```python
from build123d import *

# Parameters (mm, degrees)
SKETCH1_W           = 50
SKETCH1_H           = 40
BOSS_EXTRUDE1_DEPTH = 10
SKETCH5_W           = 6
SKETCH5_H           = 5
BOSS_EXTRUDE3_DEPTH = 10
SKETCH6_R           = 1.25
CUT_EXTRUDE1_DEPTH  = 20
SKETCH8_W           = 10
SKETCH8_H           = 40
CUT_EXTRUDE2_DEPTH  = 25
SKETCH12_W          = 5
SKETCH12_H          = 5
BOSS_EXTRUDE5_DEPTH = 10
SKETCH13_R          = 1.25
CUT_EXTRUDE4_DEPTH  = 10
SKETCH14_R          = 2.5
CUT_EXTRUDE5_DEPTH  = 10
CUT_EXTRUDE6_DEPTH  = 22
CUT_EXTRUDE7_DEPTH  = 30
CUT_EXTRUDE8_DEPTH  = 30
SCALE1_SCALE        = 2
SKETCH19_W          = 172.616714004
SKETCH19_H          = 129.336721571
SKETCH19_W_2        = 100
SKETCH19_H_2        = 80
CUT_EXTRUDE9_DEPTH  = 20
SKETCH20_W          = 100
SKETCH20_H          = 80
CUT_EXTRUDE10_DEPTH = 10
BOSS_EXTRUDE6_DEPTH = 20
SKETCH22_W          = 5
SKETCH22_H          = 10
CUT_EXTRUDE11_DEPTH = 50


with BuildPart() as part:
    # Sketch1 → Boss-Extrude1 (new body)
    with BuildSketch(Plane(origin=(669.84184187, 0, 0), x_dir=(1, 0, 0), z_dir=(0, 0, 1))):
        with Locations((-671.310344828, 437.637931034)):
            Rectangle(SKETCH1_W, SKETCH1_H)
    boss_extrude1 = extrude(amount=BOSS_EXTRUDE1_DEPTH)

    # Sketch5 → Boss-Extrude3 (add)
    with BuildSketch(Plane(origin=(23.531497042, 0, 0), x_dir=(0, 0, -1), z_dir=(1, 0, 0))):
        with Locations((-5, 442.637931034)):
            Rectangle(SKETCH5_W, SKETCH5_H)
        with Locations((-5, 432.637931034)):
            Rectangle(SKETCH5_W, SKETCH5_H)
    boss_extrude3 = extrude(amount=BOSS_EXTRUDE3_DEPTH)

    # Sketch6 → Cut-Extrude1 (cut)
    with BuildSketch(Plane(origin=(669.84184187, 445.137931034, 0), x_dir=(1, 0, 0), z_dir=(0, 1, 0))):
        with Locations(Location((-641.310344828, -5, 0), (0, 0, 180))):
            Circle(SKETCH6_R)
    cut_extrude1 = extrude(amount=-CUT_EXTRUDE1_DEPTH, mode=Mode.SUBTRACT)

    # Sketch8 → Cut-Extrude2 (cut)
    with BuildSketch(Plane.ZY.offset(26.468502958)):
        with Locations((5, 437.637931034)):
            Rectangle(SKETCH8_W, SKETCH8_H)
    extrude(amount=-CUT_EXTRUDE2_DEPTH, mode=Mode.SUBTRACT)

    # Mirror1: Boss-Extrude1, Boss-Extrude3, Cut-Extrude1 across plane
    add(boss_extrude1.mirror(Plane(origin=(-1.468502958, 0, 0), x_dir=(0, 0, 1), z_dir=(1, 0, 0))))
    add(boss_extrude3.mirror(Plane(origin=(-1.468502958, 0, 0), x_dir=(0, 0, 1), z_dir=(1, 0, 0))))
    add(cut_extrude1.mirror(Plane(origin=(-1.468502958, 0, 0), x_dir=(0, 0, 1), z_dir=(1, 0, 0))), mode=Mode.SUBTRACT)

    # Sketch12 → Boss-Extrude5 (add)
    with BuildSketch(Plane(origin=(0, 457.637931034, 0), x_dir=(1, 0, 0), z_dir=(0, 1, 0))):
        with Locations((-1.468502958, -5)):
            Rectangle(SKETCH12_W, SKETCH12_H)
    extrude(amount=BOSS_EXTRUDE5_DEPTH)

    # Sketch13 → Cut-Extrude4 (cut)
    with BuildSketch(Plane(origin=(1.031497042, 0, 0), x_dir=(0, 0, -1), z_dir=(1, 0, 0))):
        with Locations((-5, 462.637931034)):
            Circle(SKETCH13_R)
    extrude(amount=-CUT_EXTRUDE4_DEPTH, mode=Mode.SUBTRACT)

    # Sketch14 → Cut-Extrude5 (cut)
    with BuildSketch(Plane.XY.offset(10)):
        with Locations((-16.468502958, 447.637931034)):
            Circle(SKETCH14_R)
        with Locations((-16.468502958, 427.637931034)):
            Circle(SKETCH14_R)
        with Locations((13.531497042, 447.637931034)):
            Circle(SKETCH14_R)
        with Locations((13.531497042, 427.637931034)):
            Circle(SKETCH14_R)
    extrude(amount=-CUT_EXTRUDE5_DEPTH, mode=Mode.SUBTRACT)

    # Sketch15 → Cut-Extrude6 (cut)
    with BuildSketch(Plane(origin=(0, 445.137931034, 0), x_dir=(1, 0, 0), z_dir=(0, 1, 0))):
        with BuildLine():
            Line((33.531497042, -2), (28.531497042, -2))
            ThreePointArc((28.531497042, -2), (30.652817386, -2.878679656), (31.531497042, -5))
            ThreePointArc((31.531497042, -5), (30.652817386, -7.121320344), (28.531497042, -8))
            Line((28.531497042, -8), (33.531497042, -8))
            Line((33.531497042, -8), (33.531497042, -2))
        make_face()
    extrude(amount=-CUT_EXTRUDE6_DEPTH, mode=Mode.SUBTRACT)

    # Sketch17 → Cut-Extrude7 (cut)
    with BuildSketch(Plane(origin=(0, 445.137931034, 0), x_dir=(1, 0, 0), z_dir=(0, 1, 0))):
        with BuildLine():
            Line((-36.468502958, -8), (-31.468502958, -8))
            ThreePointArc((-31.468502958, -8), (-34.468502958, -5), (-31.468502958, -2))
            Line((-31.468502958, -2), (-36.468502958, -2))
            Line((-36.468502958, -2), (-36.468502958, -8))
        make_face()
    extrude(amount=-CUT_EXTRUDE7_DEPTH, mode=Mode.SUBTRACT)

    # Sketch18 → Cut-Extrude8 (cut)
    with BuildSketch(Plane(origin=(1.031497042, 0, 0), x_dir=(0, 0, -1), z_dir=(1, 0, 0))):
        with BuildLine():
            Line((-7.5, 467.637931034), (-7.5, 462.637931034))
            ThreePointArc((-7.5, 462.637931034), (-5, 465.137931034), (-2.5, 462.637931034))
            Line((-2.5, 462.637931034), (-2.5, 467.637931034))
            Line((-2.5, 467.637931034), (-7.5, 467.637931034))
        make_face()
    extrude(amount=-CUT_EXTRUDE8_DEPTH, mode=Mode.SUBTRACT)


with BuildPart() as part_1:
    # Scale1: scaled about (-1.468502958, 437.810556227, 5)
    add(part.part.scale(SCALE1_SCALE).moved(Location((1.468502958, -437.810556227, -5))))

    # Sketch19 → Cut-Extrude9 (cut)
    with BuildSketch(Plane.XY.offset(15)):
        with Locations((2.170441993, 437.623617036)):
            Rectangle(SKETCH19_W, SKETCH19_H)
        with Locations((-1.468502958, 437.465305842)):
            Rectangle(SKETCH19_W_2, SKETCH19_H_2, mode=Mode.SUBTRACT)
    extrude(amount=-CUT_EXTRUDE9_DEPTH, mode=Mode.SUBTRACT)

    # Sketch20 → Cut-Extrude10 (cut)
    with BuildSketch(Plane.XY.offset(15)):
        with Locations((-1.468502958, 437.465305842)):
            Rectangle(SKETCH20_W, SKETCH20_H)
    extrude(amount=-CUT_EXTRUDE10_DEPTH, mode=Mode.SUBTRACT)

    # Sketch21 → Boss-Extrude6 (add)
    with BuildSketch(Plane.XY.offset(5)):
        Polygon((-11.468502958, 477.465305842), (-21.468502958, 477.465305842), (-21.468502958, 397.465305842), (-11.468502958, 397.465305842), (-11.468502958, 464.619479755), align=None)
        Polygon((18.531497042, 477.465305842), (8.531497042, 477.465305842), (8.531497042, 471.588870089), (8.531497042, 397.465305842), (18.531497042, 397.465305842), align=None)
    extrude(amount=BOSS_EXTRUDE6_DEPTH)

    # Sketch22 → Cut-Extrude11 (cut)
    with BuildSketch(Plane.ZY.offset(21.468502958)):
        with Locations((17.5, 462.465305842)):
            Rectangle(SKETCH22_W, SKETCH22_H)
        with Locations((17.5, 412.465305842)):
            Rectangle(SKETCH22_W, SKETCH22_H)
    extrude(amount=-CUT_EXTRUDE11_DEPTH, mode=Mode.SUBTRACT)


solid = part_1.part
```
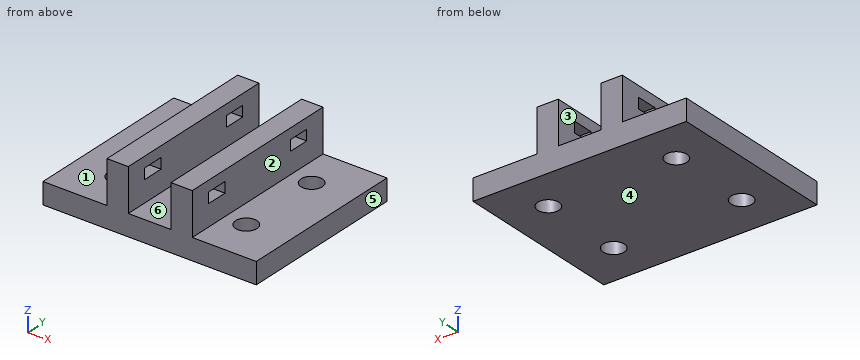
The listing builds one solid part. Answer for the finished solid, in the listing's coordinates (mm). Face numbers are marked on the shaded views. A direction names the side the tool comes from. Coordinates: 2 decimals unless noted, no trailing zeros. Order: outer loops, then holes, each group sorted by start corner. A loop starts at its lowest first (then second) coordinate and runs counter-clockwise, first axis right, second up. Notation, with made-up numbers: M 44.25,77.25 L 54.25,77.25 A24 cw 54.25,93.25 Z; hole C -14,59 d11. An arc over 180 degrees is marked long. Answer as a JSON object with one key per item and string values. Group by question number.
1. Section D-D on y = 446.5 is taken. Write down the section's boundary in (x, z).
2. Straight lines are drawn through the part: line 1 (X direction, y = 428, z = 23.5); line 2 (Z direction, x = -38.5, y = 418). For each, find the intervals that lie inside material, in ascending order.
3. Section C-C on y = 456 is taken. Write down the section's boundary in (x, z).
4. Section A-A on x = 10.5 is taken. Write down the section's boundary in (y, z), then the cut area to 3 significant figures.
5. Flat-ended cylindrical pins translate along their axes: P1, Ø16, axis at x = -5.5, y = 421, coming from the +Z side; P2, Ø1, axis at x = 7.5, y = 462.5, coming from the +Z side; P3, Ø4, axis at y = 434.5, z = 7.5, coming from the -X side; P4, Ø16, axis at y = 421, z = 15, coming from the +X side. Find the tip coordinate at first contact, or state that the pin passes through.
6. Determine the mould class of the marked faces 4, 5 and 6 for opening direction X: released by +X, released by -X, zero draft, split by the parting line, or undercut.
7. Section B-B on z = 11 is taken. Write down the section's boundary in (x, y).
8. A tool of negligible diameter and unlimited length cuts with its end or side. For the marked faces 1, 2 and 3, from which of +Z, -Z, +X, -X, +Y, -Y can it reach the whole face along a straight path? Write none if from no direction.
Values follow:
{
 "1": {"outline": "M -51.47,-5 L 48.53,-5 L 48.53,5 L 18.53,5 L 18.53,25 L 8.53,25 L 8.53,5 L -11.47,5 L -11.47,25 L -21.47,25 L -21.47,5 L -51.47,5 Z"},
 "2": {"line 1": "-21.47 to -11.47, 8.53 to 18.53", "line 2": "-5 to 5"},
 "3": {"outline": "M -51.47,-5 L -36.25,-5 L -36.25,5 L -51.47,5 Z; M -26.69,-5 L 23.75,-5 L 23.75,5 L 18.53,5 L 18.53,25 L 8.53,25 L 8.53,5 L -11.47,5 L -11.47,25 L -21.47,25 L -21.47,5 L -26.69,5 Z; M 33.31,-5 L 48.53,-5 L 48.53,5 L 33.31,5 Z"},
 "4": {"outline": "M 397.47,-5 L 477.47,-5 L 477.47,25 L 397.47,25 Z; hole M 407.47,15 L 417.47,15 L 417.47,20 L 407.47,20 Z; hole M 457.47,15 L 467.47,15 L 467.47,20 L 457.47,20 Z", "area": "2,300 mm2"},
 "5": {"P1": "z = 25", "P2": "z = 5", "P3": "x = -21.47", "P4": "x = 18.53"},
 "6": {"face 4": "zero draft", "face 5": "released by +X", "face 6": "undercut"},
 "7": {"outline": "M -21.47,397.47 L -11.47,397.47 L -11.47,477.47 L -21.47,477.47 Z; M 8.53,397.47 L 18.53,397.47 L 18.53,477.47 L 8.53,477.47 Z"},
 "8": {"face 1": "+Z, -X, +Y, -Y", "face 2": "+Z, +X, +Y, -Y", "face 3": "+Z, +Y, -Y"}
}
